Print and shaded views of the part. All mm, measured from the part's lowest x, y and z. A direction names the side the tool comes from. Round coordinates to 2 decimals unless told otherwise and drop trailing zeros. Loops run counter-clockwise (first coordinate to the right, second up) from the corner with the lowest first, then second, coordinate; pieces in that order, holes last. Notation, with made-up numbers: M 23,32.5 L 67,32.5 A14 ccw 67,53.5 Z; hole C 57,20.5 d5. An arc over 180 degrees is marked long. One line per item, written item: value. Start each with the question number.
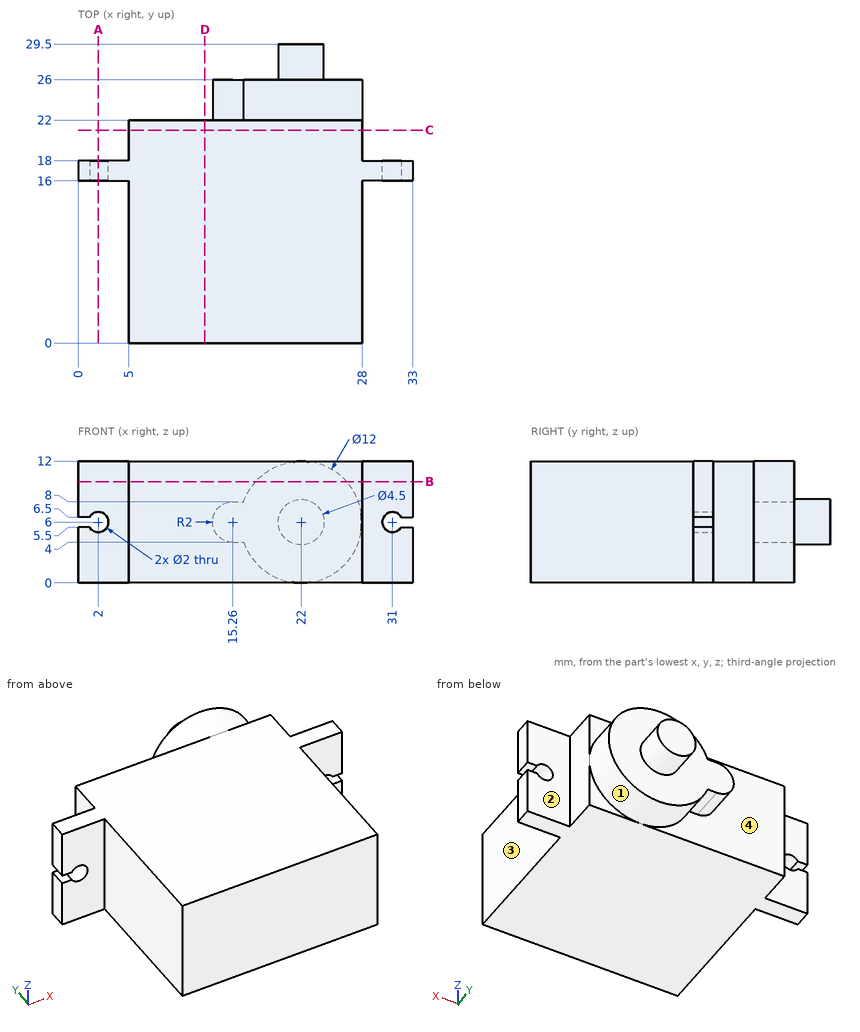
(1) Slice it at B-B, the plane z = 10. List the corners of the cut face in (x, y), and give its area (3 significant figures).
(2) Slice it at A-A, the plane x = 2. List the corners of the cut face in (y, z).
(3) Slice it at C-C, the plane y = 21. List the corners of the cut face in (x, z).
(4) Which spindle directions (+Z, -Z, +X, -X, +Y, -Y) get a long thin tool onto all of the face, cutting with end or side? Do the marked faces 1, 2, 3 and 4. Say none if no direction does.
(5) Probe L1, parallel to Z at x = 31, y = 16.55; L2, parallel to X at y = 21.5, z = 5; L3, parallel to Y at x = 22, z = 1.75. List the from-to ranges inside material, lowest first.
(6) Flat gauge pins, fed straight in: P1, Ø1, axis at x = 23, z = 6, coming from the -Y side; P2, Ø0.9, axis at x = 15.5, y = 24.5, coming from the +Z side; P3, Ø1.2, axis at y = 20, z = 3.5, coming from the -X side; P4, Ø1.5, axis at x = 31.5, z = 4, coming from the -Y side. Where does each tip first touch, or does it go through?
(7) Slice it at D-D, the plane x = 12.5. List the corners of the cut face in (y, z).
Check result:
1. outline: M 0,16 L 5,16 L 5,0 L 28,0 L 28,16 L 33,16 L 33,18 L 28,18 L 28,22 L 26.47,22 L 26.47,26 L 17.53,26 L 17.53,22 L 5,22 L 5,18 L 0,18 Z
1. area: 562 mm^2
2. outline: M 16,0 L 18,0 L 18,5 L 16,5 Z; M 16,7 L 18,7 L 18,12 L 16,12 Z
3. outline: M 5,0 L 28,0 L 28,12 L 5,12 Z
4. face 1: +Y
4. face 2: +Z, -Z, +X, +Y
4. face 3: +Z, -Z, +X, -Y
4. face 4: -X, +Y
5. L1: z = 0 to 5, 7 to 12
5. L2: x = 5 to 28
5. L3: y = 0 to 26
6. P1: stops at y = 0
6. P2: stops at z = 8
6. P3: stops at x = 5
6. P4: stops at y = 16
7. outline: M 0,0 L 22,0 L 22,12 L 0,12 Z
